Part print with two shaded views. Sizes in mm from the minimum x, y, z corner. A direction names the side the tool comes from. Coordinates: 2 decimals unless noted, no trailing zeros. Loops run counter-clockwise (first coordinate to the right, second up) from the corner with the lowest first, then second, coordinate; pieces in that order, holes last. Notation, with made-up numbers: (34, 88) -> (57, 88) arc R33 ccw to (57, 127) -> close; hole circle Ø4 at (7.25, 44). An arc over 180 degrees is marked (long way). Use one line per item in the form item = value.
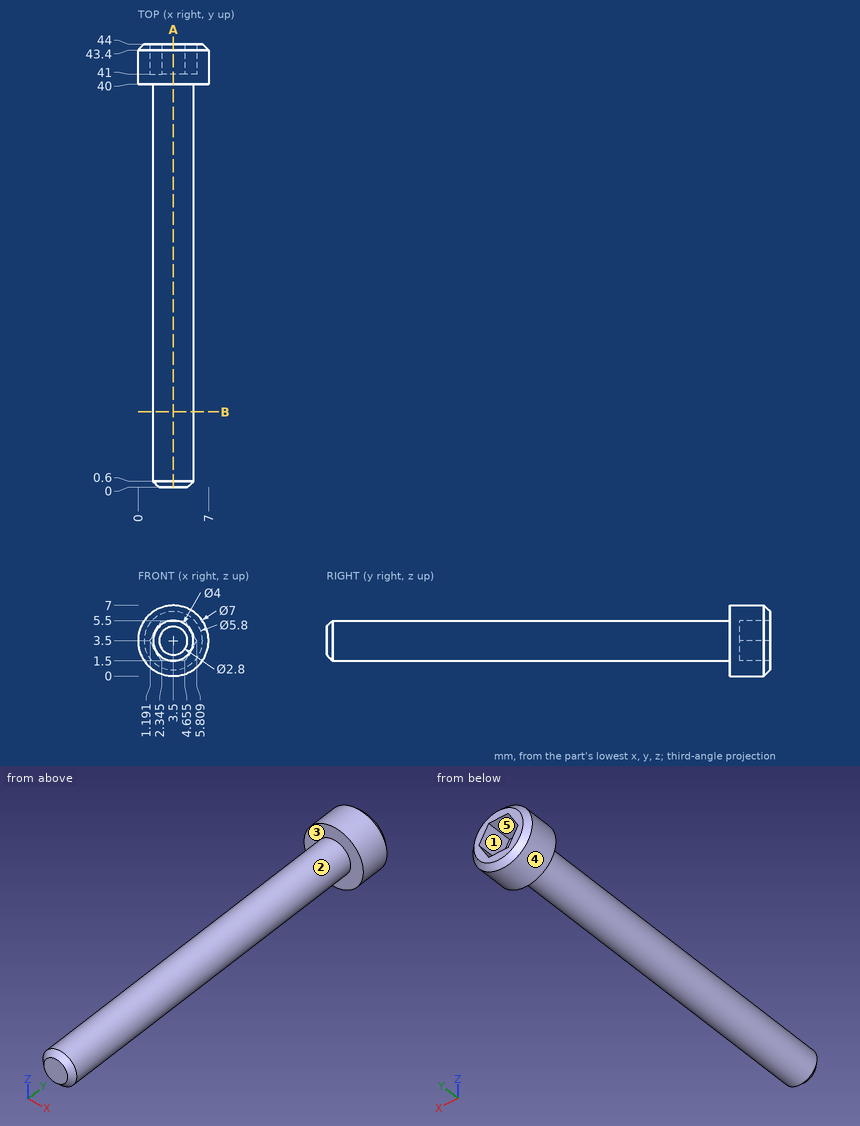
Q1. Band-saw the part on B-B, the plane y = 7.5. Write the cut outline in (x, z).
Result:
outline = circle Ø4 at (3.5, 3.5)
Q2. Band-saw the part on A-A, the plane x = 3.5. Write the cut outline in (y, z), and give its area (3 significant figures).
Result:
outline = (0, 2.1) -> (0.6, 1.5) -> (40, 1.5) -> (40, 0) -> (43.4, 0) -> (44, 0.6) -> (44, 1.5) -> (41, 1.5) -> (41, 5.5) -> (44, 5.5) -> (44, 6.4) -> (43.4, 7) -> (40, 7) -> (40, 5.5) -> (0.6, 5.5) -> (0, 4.9) -> close
area = 175 mm2
Q3. Mould opens along Z. For the marked faces 1, 2 and 3 say: released by +Z, released by -Z, zero draft, split by the parting line, or undercut.
Result:
face_1 = undercut
face_2 = split by the parting line
face_3 = zero draft
Q4. Wall check: line 1 along Y through (x, z) = (3, 2.25); line 2 along Z through (x, y) = (3.5, 41.5); line 3 along Z through (x, y) = (3.5, 28.5). Give the ranges that are in metal, low to high.
Result:
line_1 = 0 to 41
line_2 = 0 to 1.5, 5.5 to 7
line_3 = 1.5 to 5.5
Q5. Pin check, flat tips, straight feed: pin 1 Ø2 at (y, z) = (35, 6) entering from -X; pin 2 Ø2 at (y, z) = (32, 4) entering from -X; pin 3 Ø1.5 at (y, z) = (38, 2.5) entering from +X. Stop position of each tip, or through.
Result:
pin_1 = 2.18
pin_2 = 1.5
pin_3 = 5.48
Q6. Which spindle directions (+Z, -Z, +X, -X, +Y, -Y) get a long thin tool onto all of the face, cutting with end or side? Do the marked faces 4 and 5. Say none if no direction does.
Result:
face_4 = +Y, -Y
face_5 = +Y
